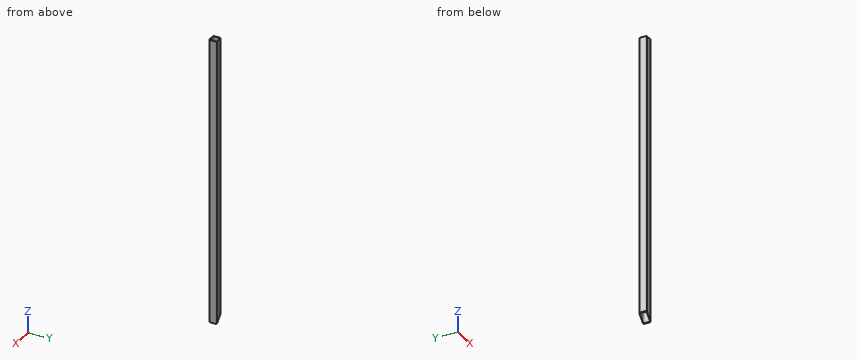
Autodesk Inventor part; units mm, degrees
ref_plane "Start plane" through (0, 0, -20) normal (0, 0, 1) x (1, 0, 0)
ref_plane "End plane" through (0, 0, 1500) normal (0, 0, 1) x (1, 0, 0)
ref_plane "Work Plane4" through (20, 0, -20) normal (-0.7071, 0, -0.7071) x (-0.7071, 0, 0.7071)
ref_plane "Start plane" through (0, 0, -20) normal (0, 0, 1) x (1, 0, 0)
ref_plane "End plane" through (0, 0, 1500) normal (0, 0, 1) x (1, 0, 0)
sketch "Sketch" plane through (0, 0, 0) normal (0, 0, 1) x (1, 0, 0)
  line L0 (-20, -16.1) -> (-20, 16.1)
  line L1 (-16.1, 20) -> (16.1, 20)
  line L2 (20, 16.1) -> (20, -16.1)
  line L3 (16.1, -20) -> (-16.1, -20)
  arc A0 (-20, -16.1) -> (-16.1, -20) centre (-16.1, -16.1) ccw
  arc A1 (-16.1, 20) -> (-20, 16.1) centre (-16.1, 16.1) ccw
  arc A2 (20, 16.1) -> (16.1, 20) centre (16.1, 16.1) ccw
  arc A3 (16.1, -20) -> (20, -16.1) centre (16.1, -16.1) ccw
  line L4 (-14.8, 17.4) -> (14.8, 17.4)
  line L5 (17.4, 14.8) -> (17.4, -14.8)
  line L6 (14.8, -17.4) -> (-14.8, -17.4)
  line L7 (-17.4, -14.8) -> (-17.4, 14.8)
  line L8 (0, 29.1308) -> (0, -29.1308) construction
  line L9 (-29.1308, 0) -> (29.1308, 0) construction
  arc A4 (-17.4, -14.8) -> (-14.8, -17.4) centre (-14.8, -14.8) ccw
  arc A5 (-14.8, 17.4) -> (-17.4, 14.8) centre (-14.8, 14.8) ccw
  arc A6 (17.4, 14.8) -> (14.8, 17.4) centre (14.8, 14.8) ccw
  arc A7 (14.8, -17.4) -> (17.4, -14.8) centre (14.8, -14.8) ccw
  dimension "d7" = 3.9
  dimension "d10" = 40
  dimension "d11" = 40
  dimension "d12" = 2.6
  dimension "d15" = 20
  dimension "d16" = 20
  dimension "d19" = 2.6
  dimension "d20" = 2.6
extrude "Body" add sketch "Sketch" along normal up to surface (1520 mm away) from surface at -20
sketch "Sketch3" plane through (0, 0, 0) normal (0, 0, 1) x (1, 0, 0)
  line L0 (0, 0) -> (10, 0)
ref_plane "Work Plane3" through (0, 0, 0) normal (0, -1, 0) x (1, 0, 0)
sketch "Sketch4" plane through (0, 0, 0) normal (0, -1, 0) x (1, 0, 0)
  line L0 (-2, -20) -> (12, -20)
  line L1 (-2, 1500) -> (12, 1500)
  dimension "d18" = 1520
ref_plane "Work Plane4" through (20, 0, -20) normal (-0.7071, 0, -0.7071) x (-0.7071, 0, 0.7071)
split "Split1" plane through (20, 0, -20) removes the side toward (-0.7071, 0, -0.7071)
equation "\"d7\" = G_IR"
equation "\"d10\" = G_H"
equation "\"d11\" = G_W"
equation "\"d12\" = G_T"
equation "\"d15\" = 0.5 * d10"
equation "\"d16\" = 0.5 * d11"
equation "\"d19\" = G_T"
equation "\"d20\" = G_T"
equation "\"d3\" = G_L"
equation "\"G_W\" = 40"
equation "\"G_H\" = 40"
equation "\"G_T\" = 2.6"
equation "\"G_IR\" = 3.9"
equation "\"G_L\" = d18"
equation "\"G_OFFSET_END\" = 0"
properties part number "EN 10210-2 - 40 x 40 x 2.6 - 1520" material "Steel, Galvanized"
Can you work these out from the model? Positions are in its coordinate system, mm. Round coordinates to 2 decimals unless told otherwise and drop trailing zeros. Loops run counter-clockwise (first coordinate to the right, second up) from the corner with the lowest first, then second, coordinate; pieces in that order, holes last. Notation, with made-up numbers: M -1,58.5 L 29,58.5 A30 cw 29,84.5 Z; hole C 62,6.25 d5. An arc over 180 degrees is marked long. Answer as a JSON object with one key per item and string values. Group by question number.
Q1. Imagine slicing it at A-A, the plane x = 4. Please give me the cut outline in (y, z).
Q2. Imagine slicing it at C-C, the plane z = 782. Please give me the cut outline in (x, y), then the cut area to 3 significant figures.
Q3. Please list where these lines run through material, in increasing order: L1, parallel to X at y = 13, z = 489.5; L2, parallel to X at y = -16.5, z = 786.
Q4. Imagine slicing it at B-B, the plane y = -2.5. Please give me the cut outline in (x, z), then the cut area to 3 significant figures.
Findings:
{
 "1": {"outline": "M -20,-4 L -17.4,-4 L -17.4,1500 L -20,1500 Z; M 17.4,-4 L 20,-4 L 20,1500 L 17.4,1500 Z"},
 "2": {"outline": "M -20,-16.1 A3.9 ccw -16.1,-20 L 16.1,-20 A3.9 ccw 20,-16.1 L 20,16.1 A3.9 ccw 16.1,20 L -16.1,20 A3.9 ccw -20,16.1 Z; hole M -17.4,-14.8 A2.6 ccw -14.8,-17.4 L 14.8,-17.4 A2.6 ccw 17.4,-14.8 L 17.4,14.8 A2.6 ccw 14.8,17.4 L -14.8,17.4 A2.6 ccw -17.4,14.8 Z", "area": "382 mm2"},
 "3": {"L1": "x = -20 to -17.4, 17.4 to 20", "L2": "x = -19.98 to -16.77, 16.77 to 19.98"},
 "4": {"outline": "M -20,20 L -17.4,17.4 L -17.4,1500 L -20,1500 Z; M 17.4,-17.4 L 20,-20 L 20,1500 L 17.4,1500 Z", "area": "7,800 mm2"}
}
